Verification items for the finished model (mm, model axes). A direction names the side the tool comes from. Round coordinates to 2 decimals unless told otherwise and drop trailing zeros. Write each loop counter-clockwise with the first axis right and the second up, starting at its lowest first coordinate (ties: lowest second). Pieces come first, ordered by that corner, then holes. Notation, with made-up numbers: (20.25, 34) -> (73.25, 34) arc R30 cw to (73.25, 63) -> close; hole circle Ø6 at (60, -9). An arc over 180 degrees is marked (long way). Answer as a JSON object with one key per item and string values. Group by question number.
(1) Scan lines: L1, parallel to Y at x = -35.5, z = 16; L2, parallel to Z at x = 31, y = -8; L3, parallel to X at y = -28.5, z = -26. Record each from-to range of solid material in increasing order. Write a range as from..to.
(2) Sectioned sample at B-B on x = 33. Record the cut outline in (y, z), and give its area (3 significant figures).
(3) Sectioned sample at D-D on x = 1. Record the cut outline in (y, z).
(4) Draft check along Z on faces 1 (the face through (32, -48.26, -25)), 2 (the face through (15.8, -48.26, -27.2)), 3 (the face through (13, -48.26, -24)), 4 (the face through (42.78, -24.4, 25.99)). Enter one of: released by +Z, released by -Z, zero draft, split by the parting line, or undercut.
(5) Set-up check for faces 5 (the face through (-1, 0, -1)), 6 (the face through (-1, -24, -30.899)): record each of +Z, -Z, +X, -X, +Y, -Y from which the full face is reachable in a straight line by a thin tool's end or side.
(6) Gauge pin test, flat end, axial feed: pin 1 Ø2 at (x, y) = (-2.5, -36.5) entering from -Z. Record the tip position at first contact, or that the pin passes through.
(7) Sectioned sample at A-A on x = -13. Record the cut outline in (y, z), and give its area (3 significant figures).
(8) Sectioned sample at C-C on y = -38.5. Record the cut outline in (x, z).
```python
from build123d import *

# Parameters (mm, degrees)
F0_W     = 88.9
F0_H     = 58.421202
F1_DEPTH = 48.26
F2_R     = 5.08
F3_W     = 5.08
F3_H     = 12.982895
F3_R     = 2.54
F3_R_2   = 4.507617
F3_R_3   = 2.893788
F4_DEPTH = 0.254


with BuildPart() as f1:
    # F0 (on Front) → F1 (new body)
    with BuildSketch(Plane.XZ):
        with Locations((-0.224516, -1.688525)):
            Rectangle(F0_W, F0_H)
    extrude(amount=F1_DEPTH)

    # F2
    f2_edges = [f1.edges().sort_by_distance(p)[0] for p in [
        (44.225484, -48.26, -1.688525),
        (-0.224516, -48.26, -30.899126),
        (44.225484, -24.13, -30.899126),
        (44.225484, 0, -1.688525),
        (44.225484, -24.13, 27.522076),
        (-0.224516, 0, 27.522076),
        (-0.224516, -48.26, 27.522076),
        (-44.674516, -24.13, 27.522076),
        (-44.674516, -24.13, -30.899126),
        (-44.674516, 0, -1.688525),
        (-0.224516, 0, -30.899126),
        (-44.674516, -48.26, -1.688525),
    ]]
    fillet(f2_edges, radius=F2_R)

    # F3 (on face) → F4 (join)
    with BuildSketch(Plane.XZ.offset(48.26)):
        with BuildLine():
            Line((-34.246631, 25.965789), (-41.732468, 25.965789))
            Line((-41.732468, 25.965789), (-41.732468, 0))
            Line((-41.732468, 0), (-34.246631, 0))
            ThreePointArc((-34.246631, 0), (-27.755184, 6.491447), (-34.246631, 12.982895))
            ThreePointArc((-34.246631, 12.982895), (-27.755184, 19.474342), (-34.246631, 25.965789))
        make_face()
        with BuildLine():
            Line((-40.462468, 2.725626), (-40.462468, 10.715656))
            Line((-40.462468, 10.715656), (-34.199979, 10.715656))
            ThreePointArc((-34.199979, 10.715656), (-30.204964, 6.720641), (-34.199979, 2.725626))
            Line((-34.199979, 2.725626), (-40.462468, 2.725626))
        make_face(mode=Mode.SUBTRACT)
        with BuildLine():
            Line((-40.462468, 15.164651), (-40.462468, 23.60866))
            Line((-40.462468, 23.60866), (-34.199979, 23.60866))
            ThreePointArc((-34.199979, 23.60866), (-29.977974, 19.386656), (-34.199979, 15.164651))
            Line((-34.199979, 15.164651), (-40.462468, 15.164651))
        make_face(mode=Mode.SUBTRACT)
        with Locations((-16.57911, 6.491447)):
            Rectangle(F3_W, F3_H)
        with Locations((-16.847532, 20.002501)):
            Circle(F3_R)
        with BuildLine():
            Line((3.091869, 13.692563), (0, 13.692563))
            Line((0, 13.692563), (0, 11.420986))
            ThreePointArc((0, 11.420986), (-11.800197, 5.710493), (0, 0))
            Line((0, 0), (0, -4.98485))
            Line((0, -4.98485), (0, -8.01362))
            ThreePointArc((0, -8.01362), (-2.492425, -10.506046), (-4.984851, -8.01362))
            Line((-4.984851, -8.01362), (-8.518415, -8.01362))
            ThreePointArc((-8.518415, -8.01362), (-2.842245, -14.072531), (3.091869, -8.266018))
            Line((3.091869, -8.266018), (3.091869, -5.489645))
            Line((3.091869, -5.489645), (3.091869, -2.965671))
            Line((3.091869, -2.965671), (3.091869, 13.692563))
        make_face()
        with Locations((-4.518354, 5.710493)):
            Circle(F3_R_2, mode=Mode.SUBTRACT)
        Polygon((7.887421, -5.994441), (7.887421, -33.247489), (11.925781, -32.99509), (11.925781, -18.356085), (15.796138, -29.466899), (19.794538, -18.356085), (19.794538, -32.99509), (25.555243, -32.99509), (25.555243, -5.994441), (19.794538, -5.994441), (15.796138, -22.386515), (11.925781, -5.994441), align=None)
        with BuildLine():
            Line((36.660735, -19.119108), (36.660735, -23.157468))
            ThreePointArc((36.660735, -23.157468), (26.694659, -25.555245), (36.660735, -27.953021))
            Line((36.660735, -27.953021), (36.660735, -30.981792))
            Line((36.660735, -30.981792), (39.689504, -30.981792))
            Line((39.689504, -30.981792), (39.689504, -19.119108))
            Line((39.689504, -19.119108), (36.660735, -19.119108))
        make_face()
        with Locations((31.966142, -25.555245)):
            Circle(F3_R_3, mode=Mode.SUBTRACT)
        with BuildLine():
            Line((36.91313, -9.02321), (36.91313, -6.751633))
            ThreePointArc((36.91313, -6.751633), (28.357434, -10.663793), (36.91313, -14.575954))
            Line((36.91313, -14.575954), (36.91313, -12.304377))
            ThreePointArc((36.91313, -12.304377), (29.806476, -10.663793), (36.91313, -9.02321))
        make_face()
    extrude(amount=F4_DEPTH)


solid = f1.part
```
Computed values:
{
 "1": {"L1": "-48.26..0", "L2": "-30.9..27.52", "L3": "-44.67..44.22"},
 "2": {"outline": "(-48.51, -30.72) -> (-48.26, -30.72) -> (-48.26, -28.26) -> (-48.51, -28.26) -> close; (-48.51, -22.85) -> (-48.26, -22.85) -> (-48.26, -25.82) arc R5.08 ccw to (-43.18, -30.9) -> (-5.08, -30.9) arc R5.08 ccw to (0, -25.82) -> (0, 22.44) arc R5.08 ccw to (-5.08, 27.52) -> (-43.18, 27.52) arc R5.08 ccw to (-48.26, 22.44) -> (-48.26, -5.52) -> (-48.51, -5.52) -> (-48.51, -6.96) -> (-48.26, -6.96) -> (-48.26, -14.37) -> (-48.51, -14.37) -> (-48.51, -15.81) -> (-48.26, -15.81) -> (-48.26, -20.39) -> (-48.51, -20.39) -> close", "area": "2,800 mm2"},
 "3": {"outline": "(-48.51, -12.73) -> (-48.26, -12.73) -> (-48.26, -25.82) arc R5.08 ccw to (-43.18, -30.9) -> (-5.08, -30.9) arc R5.08 ccw to (0, -25.82) -> (0, 22.44) arc R5.08 ccw to (-5.08, 27.52) -> (-43.18, 27.52) arc R5.08 ccw to (-48.26, 22.44) -> (-48.26, 13.69) -> (-48.51, 13.69) -> close"},
 "4": {"face 1": "undercut", "face 2": "undercut", "face 3": "zero draft", "face 4": "released by +Z"},
 "5": {"face 5": "+Z, -Z, +X, -X, +Y", "face 6": "-Z, +X, -X, +Y"},
 "6": {"pin 1": "z = -30.9"},
 "7": {"outline": "(-48.26, -25.82) arc R5.08 ccw to (-43.18, -30.9) -> (-5.08, -30.9) arc R5.08 ccw to (0, -25.82) -> (0, 22.44) arc R5.08 ccw to (-5.08, 27.52) -> (-43.18, 27.52) arc R5.08 ccw to (-48.26, 22.44) -> close", "area": "2,800 mm2"},
 "8": {"outline": "(-44.67, -25.82) arc R5.08 ccw to (-39.59, -30.9) -> (39.15, -30.9) arc R5.08 ccw to (44.23, -25.82) -> (44.23, 22.44) arc R5.08 ccw to (39.15, 27.52) -> (-39.59, 27.52) arc R5.08 ccw to (-44.67, 22.44) -> close"}
}
